Read the model definition and answer for the solid it produces. Units are mm, in the model's axes. A direction names the side the tool comes from. Round coordinates to 2 decimals unless told otherwise and drop trailing zeros. Write each loop counter-clockwise with the first axis right and the second up, starting at its lowest first coordinate (ties: lowest second). Pieces come first, ordered by that corner, then holes.
from build123d import *

# Parameters (mm, degrees)
F1_DEPTH  = 2
F2_R      = 1.5
F3_DEPTH  = 5
F4_R      = 19
F5_DEPTH  = 24
F6_W      = 47
F6_H      = 24
F7_DEPTH  = 5
F8_W      = 24
F8_H      = 5
F9_DEPTH  = 20
F11_DEPTH = 25
F12_W     = 24
F12_H     = 5
F13_DEPTH = 20
F15_DEPTH = 25
F16_R     = 4.99999


# Not quite as in the source:
# - a fillet or chamfer is up to 0.001 mm smaller than in the source, because OpenCascade refuses the exact size


with BuildPart() as f1:
    # F0 (on Front) → F1 (new body)
    with BuildSketch(Plane.XZ):
        with BuildLine():
            Line((-23.5, -23.5), (0, -23.5))
            Line((0, -23.5), (23.5, -23.5))
            Line((23.5, -23.5), (23.5, 0))
            ThreePointArc((23.5, 0), (0, 23.5), (-23.5, 0))
            Line((-23.5, 0), (-23.5, -23.5))
        make_face()
    extrude(amount=F1_DEPTH)

    # F2 (on face) → F3 (cut)
    with BuildSketch(Plane.XZ.offset(2)):
        with Locations((15.5, 0)):
            Circle(F2_R)
        with Locations((7.75, 13.4233937587)):
            Circle(F2_R)
        with Locations((-7.75, 13.4233937587)):
            Circle(F2_R)
        with Locations((-15.5, 0)):
            Circle(F2_R)
        with Locations((-7.75, -13.4233937587)):
            Circle(F2_R)
        with Locations((7.75, -13.4233937587)):
            Circle(F2_R)
        with BuildLine():
            Line((6.5, -7), (6.5, 7))
            ThreePointArc((6.5, 7), (0, 13.5), (-6.5, 7))
            Line((-6.5, 7), (-6.5, -7))
            ThreePointArc((-6.5, -7), (0, -13.5), (6.5, -7))
        make_face()
    extrude(amount=-F3_DEPTH, mode=Mode.SUBTRACT)

    # F4 (on Front) → F5 (join)
    with BuildSketch(Plane.XZ):
        with BuildLine():
            ThreePointArc((23.5, 0), (0, 23.5), (-23.5, 0))
            Line((-23.5, 0), (-23.5, -23.5))
            Line((-23.5, -23.5), (23.5, -23.5))
            Line((23.5, -23.5), (23.5, 0))
        make_face()
        with Locations((0, -0.6784388353)):
            Circle(F4_R, mode=Mode.SUBTRACT)
    extrude(amount=F5_DEPTH)

    # F6 (on face) → F7 (join)
    with BuildSketch(Plane(origin=(0, 0, -23.5), x_dir=(1, 0, 0), z_dir=(0, 0, -1))):
        with Locations((0, 12)):
            Rectangle(F6_W, F6_H)
    extrude(amount=F7_DEPTH)

    # F8 (on face) → F9 (join)
    with BuildSketch(Plane(origin=(-23.5, 0, 0), x_dir=(0, -1, 0), z_dir=(-1, 0, 0))):
        with Locations((12, -26)):
            Rectangle(F8_W, F8_H)
    extrude(amount=F9_DEPTH)

    # F10 (on face) → F11 (cut)
    with BuildSketch(Plane.XY.offset(-23.5)):
        with BuildLine():
            ThreePointArc((-32, -4), (-34.5606601718, -2.9393398282), (-33.5, -5.5))
            ThreePointArc((-33.5, -5.5), (-32.4393398282, -5.0606601718), (-32, -4))
        make_face()
        with BuildLine():
            ThreePointArc((-32, -20), (-32.4393398282, -18.9393398282), (-33.5, -18.5))
            ThreePointArc((-33.5, -18.5), (-34.5606601718, -21.0606601718), (-32, -20))
        make_face()
    extrude(amount=-F11_DEPTH, mode=Mode.SUBTRACT)

    # F12 (on face) → F13 (join)
    with BuildSketch(Plane.YZ.offset(23.5)):
        with Locations((-12, -26)):
            Rectangle(F12_W, F12_H)
    extrude(amount=F13_DEPTH)

    # F14 (on face) → F15 (cut)
    with BuildSketch(Plane.XY.offset(-23.5)):
        with BuildLine():
            ThreePointArc((35, -4), (32.4393398282, -2.9393398282), (33.5, -5.5))
            ThreePointArc((33.5, -5.5), (34.5606601718, -5.0606601718), (35, -4))
        make_face()
        with BuildLine():
            ThreePointArc((35, -20), (34.5606601718, -18.9393398282), (33.5, -18.5))
            ThreePointArc((33.5, -18.5), (32.4393398282, -21.0606601718), (35, -20))
        make_face()
    extrude(amount=-F15_DEPTH, mode=Mode.SUBTRACT)

    # F16 (radius 5 in the source; OpenCascade refuses exactly that, so slightly less here)
    f16_edges = [f1.edges().sort_by_distance(p)[0] for p in [
        (23.5, -12, -23.5),
        (43.5, -12, -23.5),
        (-23.5, -12, -23.5),
        (-43.5, -12, -23.5),
    ]]
    fillet(f16_edges, radius=F16_R)


solid = f1.part
Q1. Section B-B (z = 3.5) is taken. Determine the outline of the cut face in (x, y).
Verdict:
outline: (-23.24, -24) - (-18.53, -24) - (-18.53, -2) - (-6.5, -2) - (-6.5, 0) - (-23.24, 0) - close; (6.5, -2) - (18.53, -2) - (18.53, -24) - (23.24, -24) - (23.24, 0) - (6.5, 0) - close
Q2. Section A-A (x = -7.75) is taken. Determine the outline of the cut face in (y, z), then the cut area to 3 significant figures.
Verdict:
outline: (-24, -28.5) - (0, -28.5) - (0, -14.92) - (-2, -14.92) - (-2, -18.03) - (-24, -18.03) - close; (-24, 16.67) - (-2, 16.67) - (-2, 14.92) - (0, 14.92) - (0, 22.19) - (-24, 22.19) - close; (-2, -11.92) - (0, -11.92) - (0, 11.92) - (-2, 11.92) - close
area: 441 mm2
Q3. Straight lines are drawn through the part: probe 1 along Y at (x, z) = (33.5, -25.35); probe 2 along Z at (x, y) = (-7.75, -0.95); probe 3 along Y at (x, z) = (-32.5, -26). For each, find the intervals that lie inside material, in ascending order.
Verdict:
probe 1: y = -24 to -21.5, -18.5 to -5.5, -2.5 to 0
probe 2: z = -28.5 to -14.92, -11.92 to 11.92, 14.92 to 22.19
probe 3: y = -24 to -21.12, -18.88 to -5.12, -2.88 to 0
Q4. Flat-ended cylindrical pins translate along their axes: pin 1 Ø11 at (x, y) = (-32, -6) entering from +Z; pin 2 Ø11.5 at (x, z) = (-3, 4) entering from -Y; pin 3 Ø2 at (y, z) = (-14, -8) entering from -X; pin 4 Ø2.5 at (x, z) = (-7.75, 13.42) entering from +Y. Find the tip coordinate at first contact, or state that the pin passes through.
Verdict:
pin 1: stops at z = -23.08
pin 2: stops at y = -2
pin 3: stops at x = -23.5
pin 4: passes through
Q5. Section D-D (x = 15.5) is taken. Determine the outline of the cut face in (y, z), then the cut area to 3 significant figures.
Verdict:
outline: (-24, -28.5) - (0, -28.5) - (0, -1.5) - (-2, -1.5) - (-2, -11.67) - (-24, -11.67) - close; (-24, 10.31) - (-2, 10.31) - (-2, 1.5) - (0, 1.5) - (0, 17.66) - (-24, 17.66) - close
area: 618 mm2
Q6. Which of the six approach directions +Z, -Z, +X, -X, +Y, -Y give full straight-line access (tool end or side, diameter ignored) to faces 1 (the flat face through (-33, -12, -23.5)), 2 (the flat face through (23.5, -12, -9)), 3 (the cylindrical face through (-0.1, -1, -13.5))?
Verdict:
face 1: +Z, -X, +Y, -Y
face 2: +Z, +X, +Y, -Y
face 3: +Y, -Y
Q7. Determine the mould class of faces 4 (the cylindrical face through (42.07, -11.83, -25)), 5 (the flat face through (33, -12, -23.5)), 6 (the cylindrical face through (6.56, -1.014, -14.336)) for opening direction X: pulls with the +X half, pulls with the -X half, needs draft (parallel to the pull), parting line crosses it, or undercut.
Verdict:
face 4: pulls with the +X half
face 5: needs draft
face 6: undercut
